Input: part model. Units: mm. Frame: model coordinates. A direction names the side the tool comes from. Give positions to 0.01 mm unless a question says otherwise; leave off trailing zeros. Loops run counter-clockwise (first coordinate to the right, second up) from the corner with the lowest first, then second, coordinate; pieces in that order, holes last. Notation, with made-up numbers: M -20,-36.75 L 1,-36.75 A22 cw 1,-23.75 Z; hole C -14.75,-29.5 d5. An arc over 180 degrees is marked long. Answer as a JSON object with one key per item and string values. Group by question number.
1) Ray query, L1, parallel to Y at x = 19, z = 22.5; L2, parallel to X at y = 6.5, z = 3; L3, parallel to X at y = 8, z = 11.5. Return the intervals inside material, ascending.
2) Section query C-C on y = 11.5. Count the separate pieces of the cut face and the enclosed holes in it, plus the area to 3 significant figures.
3) Section query D-D on z = 30. Return loops of the section in (x, y) (3 decimals), plus the area to 3 significant figures.
4) Draft query along Z for faces 4 (the flat face through (-20, 14, -15.5)), 5 (the cylindrical face through (-38.952, 7.395, -11.919)), 6 (the flat face through (0, 13, 13)), 7 (the flat face through (47, 14, 0)). Return one class per face: +Z half, -Z half, draft (parallel to the pull), parting line (faces both ways), or undercut.
5) First-contact query: P1, Ø8, axis at y = 10.5, z = 10, coming from the -X side; P2, Ø1.6, axis at y = 14, z = 21, coming from the -X side; P3, Ø5.5, axis at x = -15, z = -10.5, coming from the +Y side. Flat tips, straight axial feed; report the tip coordinate or a pass-through.
6) Section query B-B on x = -40.5. Return loops of the section in (y, z).
7) Access query for faces 1 (the cylindrical face through (0.133, 7.395, -1.016)), 2 (the flat face through (1.75, 14, 21)), 3 (the flat face through (20, 14, -15.5)). Directions: +Z, -Z, +X, -X, +Y, -Y. A direction counts if a zero-diameter tool reaches every point of the face in a straight line with its end or side. Return the directions, or none.
8) Section query A-A on z = 13. Return loops of the section in (x, y).
from build123d import *

# Parameters (mm, degrees)
BOSS_EXTRUDE1_DEPTH      = 15
CUT_EXTRUDE1_DEPTH       = 2
M2_5X0_45_TAPPED_HOLE1_D = 2.05
CUT_EXTRUDE2_START       = -2
SKETCH9_W                = 25
SKETCH9_H                = 2
CUT_EXTRUDE2_DEPTH       = 2
M5X0_8_TAPPED_HOLE1_D    = 4.2


with BuildPart() as part:
    # Sketch1 → Boss-Extrude1 (new body)
    with BuildSketch(Plane(origin=(0, 0, 0), x_dir=(1, 0, 0), z_dir=(0, 1, 0))):
        with BuildLine():
            Line((-47.5, 17.5), (47.5, 17.5))
            Line((47.5, 17.5), (47.5, 0))
            ThreePointArc((47.5, 0), (33.587572106, -33.587572106), (0, -47.5))
            ThreePointArc((0, -47.5), (-33.587572106, -33.587572106), (-47.5, 0))
            Line((-47.5, 0), (-47.5, 17.5))
        make_face()
    extrude(amount=BOSS_EXTRUDE1_DEPTH)

    # Sketch2 → Cut-Extrude1 (cut)
    with BuildSketch(Plane(origin=(0, 15, 0), x_dir=(1, 0, 0), z_dir=(0, 1, 0))):
        with BuildLine():
            Line((13.71356205, -21.139861194), (1.75, -18.14509732))
            Line((1.75, -18.14509732), (1.75, -22.707023927))
            Line((1.75, -22.707023927), (1.75, -24.707023927))
            ThreePointArc((1.75, -24.707023927), (0, -24.425226847), (-1.75, -24.707023927))
            Line((-1.75, -24.707023927), (-1.75, -22.707023927))
            Line((-1.75, -22.707023927), (-1.75, -18.14509732))
            Line((-1.75, -18.14509732), (-13.71356205, -21.139861194))
            Line((-13.71356205, -21.139861194), (-15.653699161, -21.625523616))
            ThreePointArc((-15.653699161, -21.625523616), (-15.805291295, -19.859474518), (-16.503608401, -18.230283671))
            Line((-16.503608401, -18.230283671), (-14.56347129, -17.744621249))
            Line((-14.56347129, -17.744621249), (-3.599185624, -15))
            Line((-3.599185624, -15), (-24.237297726, -4.800131508))
            Line((-24.237297726, -4.800131508), (-26.03027479, -3.913997633))
            ThreePointArc((-26.03027479, -3.913997633), (-25.002279798, -2.469997671), (-24.479540508, -0.77628777))
            Line((-24.479540508, -0.77628777), (-22.686563443, -1.662421645))
            Line((-22.686563443, -1.662421645), (-1.893248081, -11.93899545))
            Line((-1.893248081, -11.93899545), (-1.75, -11.85490268))
            Line((-1.75, -11.85490268), (-1.75, -7.292976073))
            Line((-1.75, -7.292976073), (-1.75, -5.292976073))
            ThreePointArc((-1.75, -5.292976073), (0, -5.574773153), (1.75, -5.292976073))
            Line((1.75, -5.292976073), (1.75, -7.292976073))
            Line((1.75, -7.292976073), (1.75, -11.85490268))
            Line((1.75, -11.85490268), (1.893248081, -11.93899545))
            Line((1.893248081, -11.93899545), (22.686563443, -1.662421645))
            Line((22.686563443, -1.662421645), (24.479540508, -0.77628777))
            ThreePointArc((24.479540508, -0.77628777), (25.002279798, -2.469997671), (26.03027479, -3.913997633))
            Line((26.03027479, -3.913997633), (24.237297726, -4.800131508))
            Line((24.237297726, -4.800131508), (3.599185624, -15))
            Line((3.599185624, -15), (14.56347129, -17.744621249))
            Line((14.56347129, -17.744621249), (16.503608401, -18.230283671))
            ThreePointArc((16.503608401, -18.230283671), (15.805291295, -19.859474518), (15.653699161, -21.625523616))
            Line((15.653699161, -21.625523616), (13.71356205, -21.139861194))
        make_face()
    extrude(amount=-CUT_EXTRUDE1_DEPTH, mode=Mode.SUBTRACT)

    # M2.5x0.45 Tapped Hole1 (through all)
    with Locations(Plane(origin=(0, 15, 0), x_dir=(1, 0, 0), z_dir=(0, 1, 0))):
        with Locations((-30, 0), (0, 0), (30, 0), (21.213203436, -21.213203436), (0, -30), (-21.213203436, -21.213203436)):
            Hole(M2_5X0_45_TAPPED_HOLE1_D / 2)

    # Sketch9 → Cut-Extrude2 (cut)
    with BuildSketch(Plane(origin=(0, 15, 0), x_dir=(1, 0, 0), z_dir=(0, 1, 0)).offset(CUT_EXTRUDE2_START)):
        with Locations((-20, 16.5)):
            Rectangle(SKETCH9_W, SKETCH9_H)
        with Locations((20, 16.5)):
            Rectangle(SKETCH9_W, SKETCH9_H)
        with BuildLine():
            Line((11.776266552, -43.949625096), (12.293904642, -45.881476749))
            ThreePointArc((12.293904642, -45.881476749), (37.684283664, -28.916167878), (47.5, 0))
            Line((47.5, 0), (45.5, 0))
            ThreePointArc((45.5, 0), (36.097576983, -27.69864502), (11.776266552, -43.949625096))
        make_face()
        with BuildLine():
            Line((-47.5, 0), (-45.5, 0))
            ThreePointArc((-45.5, 0), (-36.097576983, -27.69864502), (-11.776266552, -43.949625096))
            Line((-11.776266552, -43.949625096), (-12.293904642, -45.881476749))
            ThreePointArc((-12.293904642, -45.881476749), (-37.684283664, -28.916167878), (-47.5, 0))
        make_face()
    extrude(amount=CUT_EXTRUDE2_DEPTH, mode=Mode.SUBTRACT)

    # M5x0.8 Tapped Hole1 (through all)
    with Locations(Plane(origin=(0, 15, 0), x_dir=(1, 0, 0), z_dir=(0, 1, 0))):
        with Locations((-40.5, 10.5), (-34.183542703, -14.159286998), (34.183542703, -14.159286998), (-14.159286998, -34.183542703), (14.159286998, -34.183542703), (40.5, 10.5), (-15, 10.5), (15, 10.5)):
            Hole(M5X0_8_TAPPED_HOLE1_D / 2)

    # Sketch15 → Revolve2 (revolve)
    with BuildSketch(Plane(origin=(0, 0, 0), x_dir=(0, 0, -1), z_dir=(1, 0, 0))):
        with BuildLine():
            Line((-43, 17.4746), (-43, 15))
            Line((-43, 15), (-40.5254, 15))
            ThreePointArc((-40.5254, 15), (-41.250193559, 16.749806441), (-43, 17.4746))
        make_face()
    revolve(axis=Axis((0, 15, 43), (0, 1, 0)))

    # Sketch17 → Revolve3 (revolve)
    with BuildSketch(Plane(origin=(0, 0, 0), x_dir=(0, 0, -1), z_dir=(1, 0, 0))):
        with BuildLine():
            Line((14.9746, 15), (12.5, 15))
            Line((12.5, 15), (12.5, 17.4746))
            ThreePointArc((12.5, 17.4746), (14.249806441, 16.749806441), (14.9746, 15))
        make_face()
    revolve(axis=Axis((0, 15, -12.5), (0, 1, 0)))


solid = part.part
Output:
{
 "1": {"L1": "y = 0 to 15", "L2": "x = -47.41 to 47.41", "L3": "x = -46.09 to 46.09"},
 "2": {"separate pieces": "1", "enclosed holes": "14", "area": "5,080 mm^2"},
 "3": {"outline": "M -36.827,0 L -1.025,0 L -1.025,15 L -34.209,15 L -34.209,13 L -36.827,13 Z; M 1.025,0 L 36.827,0 L 36.827,13 L 34.209,13 L 34.209,15 L 1.025,15 Z", "area": "1,060 mm^2"},
 "4": {"face 4": "-Z half", "face 5": "undercut", "face 6": "undercut", "face 7": "+Z half"},
 "5": {"P1": "stops at x = -47.12", "P2": "stops at x = -40.77", "P3": "stops at y = 15"},
 "6": {"outline": "M 0,-17.5 L 15,-17.5 L 15,-12.6 L 0,-12.6 Z; M 0,-8.4 L 15,-8.4 L 15,20.74 L 13,20.74 L 13,24.82 L 0,24.82 Z"},
 "7": {"face 1": "+Y, -Y", "face 2": "+Y", "face 3": "-Z, +Y"},
 "8": {"outline": "M -45.69,0 L -35.93,0 L -35.93,15 L -43.6,15 L -43.6,13 L -45.69,13 Z; M -32.43,0 L 32.43,0 L 32.43,15 L 7.65,15 L 7.65,13 L -7.65,13 L -7.65,15 L -32.43,15 Z; M 35.93,0 L 45.69,0 L 45.69,13 L 43.6,13 L 43.6,15 L 35.93,15 Z"}
}
